```python
from build123d import *

# Parameters (mm, degrees)
SKETCH2_R           = 0.889
BOSS_EXTRUDE1_DEPTH = 0.65


with BuildPart() as part:
    # Sketch2 → Boss-Extrude1 (new body)
    with BuildSketch(Plane.XY.offset(0.635)):
        with BuildLine():
            Line((23.8125, 8.636), (-23.8125, 8.636))
            ThreePointArc((-23.8125, 8.636), (-26.237169153, 7.631669153), (-27.2415, 5.207))
            Line((-27.2415, 5.207), (-27.2415, -5.207))
            ThreePointArc((-27.2415, -5.207), (-26.237169153, -7.631669153), (-23.8125, -8.636))
            Line((-23.8125, -8.636), (23.8125, -8.636))
            ThreePointArc((23.8125, -8.636), (26.237169153, -7.631669153), (27.2415, -5.207))
            Line((27.2415, -5.207), (27.2415, 5.207))
            ThreePointArc((27.2415, 5.207), (26.237169153, 7.631669153), (23.8125, 8.636))
        make_face()
        with Locations((-25.223, 0)):
            Circle(SKETCH2_R, mode=Mode.SUBTRACT)
        with Locations((25.223, 0)):
            Circle(SKETCH2_R, mode=Mode.SUBTRACT)
        with BuildLine():
            Line((23.5855, -2.470494747), (23.5855, 2.470494747))
            ThreePointArc((23.5855, 2.470494747), (23.734063659, 2.866942592), (24.10658046, 3.068122331))
            ThreePointArc((24.10658046, 3.068122331), (25.966463543, 5.354384043), (23.8125, 7.366))
            Line((23.8125, 7.366), (-23.8125, 7.366))
            ThreePointArc((-23.8125, 7.366), (-25.966463543, 5.354384043), (-24.10658046, 3.068122331))
            ThreePointArc((-24.10658046, 3.068122331), (-23.734063659, 2.866942592), (-23.5855, 2.470494747))
            Line((-23.5855, 2.470494747), (-23.5855, -2.470494747))
            ThreePointArc((-23.5855, -2.470494747), (-23.734063659, -2.866942592), (-24.10658046, -3.068122331))
            ThreePointArc((-24.10658046, -3.068122331), (-25.966463543, -5.354384043), (-23.8125, -7.366))
            Line((-23.8125, -7.366), (23.8125, -7.366))
            ThreePointArc((23.8125, -7.366), (25.966463543, -5.354384043), (24.10658046, -3.068122331))
            ThreePointArc((24.10658046, -3.068122331), (23.734063659, -2.866942592), (23.5855, -2.470494747))
        make_face(mode=Mode.SUBTRACT)
    extrude(amount=BOSS_EXTRUDE1_DEPTH)


solid = part.part
```
Build history of the part. All positions in model axes, mm. A direction names the side the tool comes from. Give positions to 0.01 mm unless a question says otherwise; leave off trailing zeros. Loops run counter-clockwise (first coordinate to the right, second up) from the corner with the lowest first, then second, coordinate; pieces in that order, holes last.
1) Two-plate mould, pull along Y, no slides. Class faces 1 (the face through (0, -8, 0.635)), 2 (the face through (-26.264, -7.605, 0.955)), 3 (the face through (-25.97, -5.31, 0.96)): released by +Y, released by -Y, zero draft, split by the parting line, or undercut.
Values follow:
face 1: zero draft
face 2: released by -Y
face 3: undercut
2) Band-saw the part on C-C on x = -9. List the corners of the cut face in (y, z) (3 decimals), then the cut area to 3 significant figures.
Values follow:
outline: (-8.636, 0.635) - (-7.366, 0.635) - (-7.366, 1.285) - (-8.636, 1.285) - close; (7.366, 0.635) - (8.636, 0.635) - (8.636, 1.285) - (7.366, 1.285) - close
area: 1.65 mm2
3) Probe line 1 along Y through (x, z) = (-9, 0.8); line 2 along X through (y, z) = (-1.25, 1.1); line 3 along X through (y, z) = (-6.25, 1). List the from-to ranges inside material, lowest first.
Values follow:
line 1: y = -8.64 to -7.37, 7.37 to 8.64
line 2: x = -27.24 to -23.59, 23.59 to 27.24
line 3: x = -27.08 to -25.7, 25.7 to 27.08
4) 3-axis set-ups, long thin cutter, end or side, ignore diameter. For faces 4 (the face through (26.21, -7.66, 0.96)), 5 (the face through (25.963, -5.4, 0.955)): which of +Z, -Z, +X, -X, +Y, -Y reach the whole face in a straight line?
Values follow:
face 4: +Z, -Z, +X, -Y
face 5: +Z, -Z
5) Band-saw the part on D-D on y = 4. List the corners of the cut face in (x, z) (1 decimal).
Values follow:
outline: (-27.2, 0.6) - (-25.6, 0.6) - (-25.6, 1.3) - (-27.2, 1.3) - close; (25.6, 0.6) - (27.2, 0.6) - (27.2, 1.3) - (25.6, 1.3) - close
6) Drop a flat-ended pin along its axis: P1, Ø10, axis at x = 15.5, y = 5, coming from the -Z side (3 decimals). Give the stop position or say it passes through.
Values follow:
P1: stops at z = 0.635
7) Band-saw the part on B-B on z = 0.9. List the corners of the cut face in (x, y), then the cut area to 3 significant figures.
Values follow:
outline: (-27.24, -5.21) arc R3.43 ccw to (-23.81, -8.64) - (23.81, -8.64) arc R3.43 ccw to (27.24, -5.21) - (27.24, 5.21) arc R3.43 ccw to (23.81, 8.64) - (-23.81, 8.64) arc R3.43 ccw to (-27.24, 5.21) - close; hole circle Ø1.78 at (-25.22, 0); hole (-24.11, -3.07) arc R2.16 ccw to (-23.81, -7.37) - (23.81, -7.37) arc R2.16 ccw to (24.11, -3.07) arc R0.6 cw to (23.59, -2.47) - (23.59, 2.47) arc R0.6 cw to (24.11, 3.07) arc R2.16 ccw to (23.81, 7.37) - (-23.81, 7.37) arc R2.16 ccw to (-24.11, 3.07) arc R0.6 cw to (-23.59, 2.47) - (-23.59, -2.47) arc R0.6 cw to start; hole circle Ø1.78 at (25.22, 0)
area: 198 mm2
8) Band-saw the part on A-A on y = 0. List the corners of the cut face in (x, z) (1 decimal), then the cut area to 3 significant figures.
Values follow:
outline: (-27.2, 0.6) - (-26.1, 0.6) - (-26.1, 1.3) - (-27.2, 1.3) - close; (-24.3, 0.6) - (-23.6, 0.6) - (-23.6, 1.3) - (-24.3, 1.3) - close; (23.6, 0.6) - (24.3, 0.6) - (24.3, 1.3) - (23.6, 1.3) - close; (26.1, 0.6) - (27.2, 0.6) - (27.2, 1.3) - (26.1, 1.3) - close
area: 2.44 mm2
